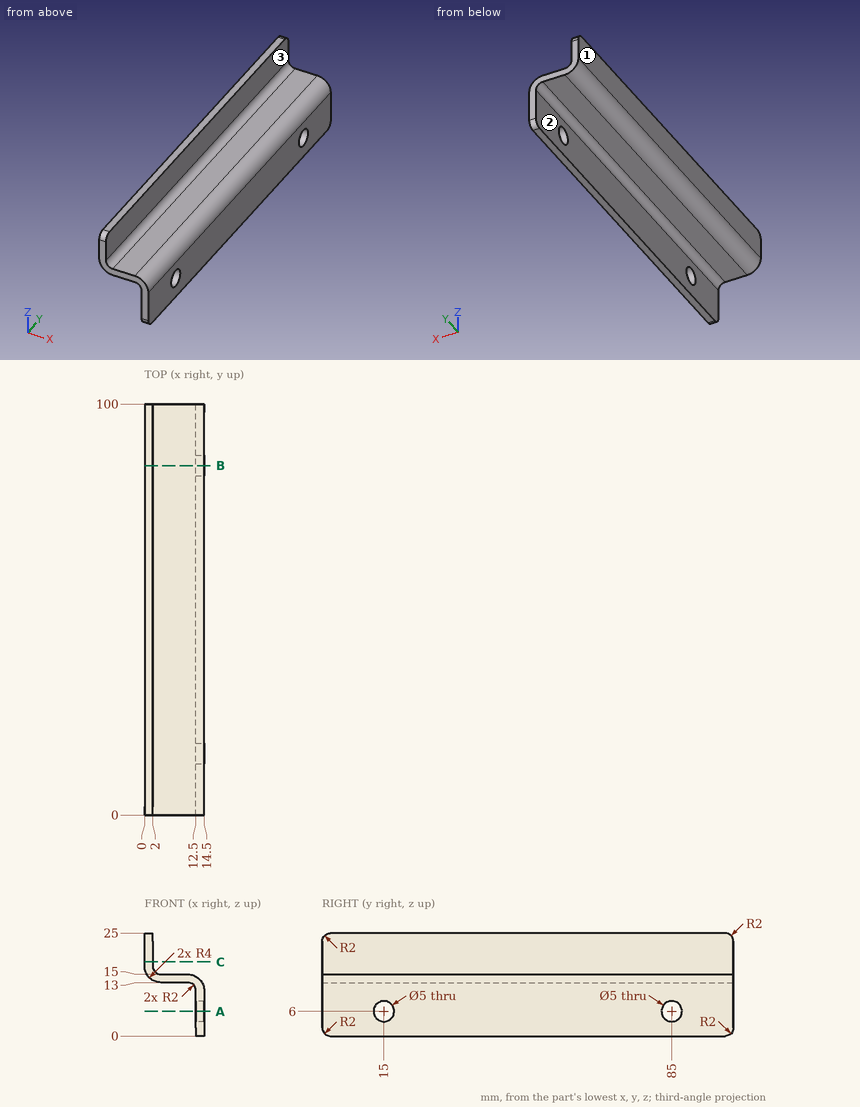
Answer from the drawing. Dimensions are ordinates in mm from the lowest x, y and z of the part. A direction names the side the tool comes from. Coordinates: 2 decimals unless noted, no trailing zeros. Order: outer loops, then holes, each group sorted by start corner. A loop starts at its lowest first (then second) coordinate and runs counter-clockwise, first axis right, second up. Notation, with made-up numbers: (59, 16.5) -> (81, 16.5) arc R21 ccw to (81, 30.5) -> close; hole circle Ø1 at (66, 65). An arc over 180 degrees is marked (long way). Answer as a JSON object with one key per item and string values.
1) A cutting plane is placed at C-C, the plane z = 18. Determine the outline of the cut face in (x, y).
Model answer:
{"outline": "(0, 0) -> (2, 0) -> (2, 100) -> (0, 100) -> close"}
2) A cutting plane is placed at B-B, the plane y = 85. Determine the outline of the cut face in (x, z).
Model answer:
{"outline": "(0, 17) arc R4 ccw to (4, 13) -> (10.5, 13) arc R2 cw to (12.5, 11) -> (12.5, 8.5) -> (14.5, 8.5) -> (14.5, 11) arc R4 ccw to (10.5, 15) -> (4, 15) arc R2 cw to (2, 17) -> (2, 25) -> (0, 25) -> close; (12.5, 0) -> (14.5, 0) -> (14.5, 3.5) -> (12.5, 3.5) -> close"}
3) Consider line 1 along Y through (x, z) = (13.95, 6); line 2 along Z through (x, y) = (5, 5); line 3 along X through (y, z) = (58.5, 23.5). Determine where each line is inside the solid, lowest interval first. Write a range as from..to.
Model answer:
{"line 1": "y = 0..12.5, 17.5..82.5, 87.5..100", "line 2": "z = 13..15", "line 3": "x = 0..2"}
4) A tool of negligible diameter and unlimited length cuts with its end or side. For the marked faces 1, 2 and 3, from which of +Z, -Z, +X, -X, +Y, -Y can it reach the whole face along a straight path? Write none if from no direction.
Model answer:
{"face 1": "+Z, -Z, -X, +Y, -Y", "face 2": "-Z, -X, +Y, -Y", "face 3": "+Z, +X, +Y, -Y"}
5) A cutting plane is placed at A-A, the plane z = 6. Determine the outline of the cut face in (x, y), plus the area to 3 significant figures.
Model answer:
{"outline": "(12.5, 0) -> (14.5, 0) -> (14.5, 12.5) -> (12.5, 12.5) -> close; (12.5, 17.5) -> (14.5, 17.5) -> (14.5, 82.5) -> (12.5, 82.5) -> close; (12.5, 87.5) -> (14.5, 87.5) -> (14.5, 100) -> (12.5, 100) -> close", "area": "180 mm²"}
6) Each of these flat-tipped pins is pushed along its axis until it touches: pin 1 (12 mm diameter, centred on y = 60.5, z = 3, fed in from -X); pin 2 (5 mm diameter, centred on x = 7.5, y = 21.5, fed in from +Z); pin 3 (2 mm diameter, centred on x = 6.5, y = 67.5, fed in from -Z); pin 4 (8 mm diameter, centred on y = 15, z = 6, fed in from +X). Where does it stop, or does it pass through?
Model answer:
{"pin 1": "stops at x = 12.5", "pin 2": "stops at z = 15", "pin 3": "stops at z = 13", "pin 4": "stops at x = 14.5"}
